Source: CAD feature listing. Evaluate the final solid. Frame: model axes, mm. Face numbers are marked on the shaded views. A direction names the side the tool comes from. Round coordinates to 2 decimals unless told otherwise and drop trailing zeros. Write each loop counter-clockwise with the first axis right and the second up, starting at its lowest first coordinate (ties: lowest second). Pieces come first, ordered by that corner, then holes.
from build123d import *

# Parameters (mm, degrees)
SKETCH_1_R          = 1.5
EXTRUDE_1_DEPTH     = 1.8
EXTRUDE_2_DEPTH     = 2
SKETCH_3_W          = 7.75
SKETCH_3_H          = 0.5
CUT_EXTRUDE_1_DEPTH = 20.686607123


with BuildPart() as part:
    # 草图1 → 凸台-拉伸1 (new body)
    with BuildSketch(Plane.XY):
        with BuildLine():
            Line((-9.503288904, -4.75), (-19, -4.75))
            Line((-19, -4.75), (-19, 4.75))
            Line((-19, 4.75), (19, 4.75))
            Line((19, 4.75), (19, -4.75))
            Line((19, -4.75), (9.503288904, -4.75))
            ThreePointArc((9.503288904, -4.75), (0, -0.5), (-9.503288904, -4.75))
        make_face()
        with Locations((-16, 0.25)):
            Circle(SKETCH_1_R, mode=Mode.SUBTRACT)
        with Locations((16, 0.25)):
            Circle(SKETCH_1_R, mode=Mode.SUBTRACT)
    extrude(amount=EXTRUDE_1_DEPTH)

    # 草图2 → 凸台-拉伸2 (add)
    with BuildSketch(Plane.XY.offset(1.8)):
        with BuildLine():
            Line((-11.25, 4.75), (-11.25, -4.75))
            Line((-11.25, -4.75), (-9.503288904, -4.75))
            ThreePointArc((-9.503288904, -4.75), (0, -0.5), (9.503288904, -4.75))
            Line((9.503288904, -4.75), (11.25, -4.75))
            Line((11.25, -4.75), (11.25, 4.75))
            Line((11.25, 4.75), (-11.25, 4.75))
        make_face()
    extrude(amount=EXTRUDE_2_DEPTH)

    # 草图3 → 切除-拉伸1 (cut, through all)
    with BuildSketch(Plane.XY.offset(1.8)):
        with Locations((-15.125, -4.5)):
            Rectangle(SKETCH_3_W, SKETCH_3_H)
        with Locations((15.125, -4.5)):
            Rectangle(SKETCH_3_W, SKETCH_3_H)
    extrude(amount=-CUT_EXTRUDE_1_DEPTH, mode=Mode.SUBTRACT)


solid = part.part
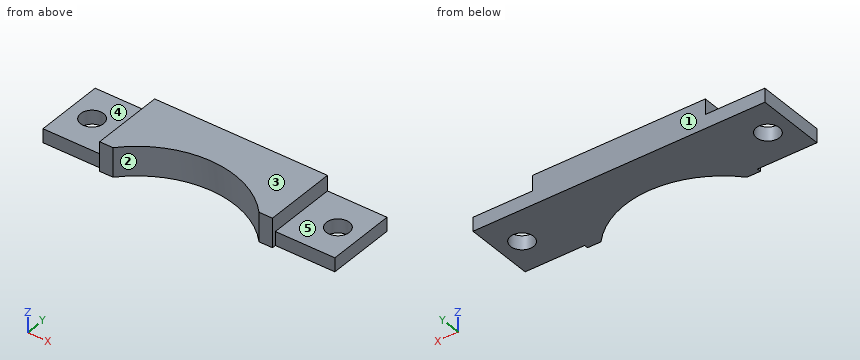
1) Contact query for flat-ended pins moving along their axis: P1, Ø2, axis at x = 14, z = 1, coming from the -Y side; P2, Ø4, axis at x = 17, y = -0.5, coming from the +Z side; P3, Ø1.1, axis at y = 1.5, z = 2.5, coming from the +X side. Output: stop coordinate, or through.
Taken from the geometry:
P1: stops at y = -4.25
P2: stops at z = 1.8
P3: stops at x = 11.25
2) Section query D-D on y = -3.5. Return the cut outline in (x, z).
Taken from the geometry:
outline: (-19, 0) - (-8.22, 0) - (-8.22, 3.8) - (-11.25, 3.8) - (-11.25, 1.8) - (-19, 1.8) - close; (8.22, 0) - (19, 0) - (19, 1.8) - (11.25, 1.8) - (11.25, 3.8) - (8.22, 3.8) - close
3) Section query C-C on z = 0.35. Return the cut outline in (x, y), then the cut area to 3 significant figures.
Taken from the geometry:
outline: (-19, -4.25) - (-11.25, -4.25) - (-11.25, -4.75) - (-9.5, -4.75) arc R12.75 cw to (9.5, -4.75) - (11.25, -4.75) - (11.25, -4.25) - (19, -4.25) - (19, 4.75) - (-19, 4.75) - close; hole circle Ø3 at (-16, 0.25); hole circle Ø3 at (16, 0.25)
area: 283 mm2
4) Section query A-A on y = 0.25. Return the cut outline in (x, z).
Taken from the geometry:
outline: (-19, 0) - (-17.5, 0) - (-17.5, 1.8) - (-19, 1.8) - close; (-14.5, 0) - (14.5, 0) - (14.5, 1.8) - (11.25, 1.8) - (11.25, 3.8) - (-11.25, 3.8) - (-11.25, 1.8) - (-14.5, 1.8) - close; (17.5, 0) - (19, 0) - (19, 1.8) - (17.5, 1.8) - close
5) Pull-direction query (X, two-part tool) for the marked faces 1 and 2; classes: released by +X, released by -X, zero draft, split by the parting line, or undercut.
Taken from the geometry:
face 1: zero draft
face 2: undercut
6) Material intervals for line 1 (Y direction, x = 16, z = 1.4); line 2 (X direction, y = -2.25, z = 0.25); line 3 (Z direction, x = 15, y = -1.25), sorted ascending.
Taken from the geometry:
line 1: y = -4.25 to -1.25, 1.75 to 4.75
line 2: x = -19 to -6.45, 6.45 to 19
line 3: z = 0 to 1.8
7) Section query B-B on x = 15.5. Return the cut outline in (y, z).
Taken from the geometry:
outline: (-4.25, 0) - (-1.16, 0) - (-1.16, 1.8) - (-4.25, 1.8) - close; (1.66, 0) - (4.75, 0) - (4.75, 1.8) - (1.66, 1.8) - close
8) Reachability of the marked faces 3, 4 and 5 from +Z, -Z, +X, -X, +Y, -Y: full face, straight path, thin tool, end or side. Return the list, or none.
Taken from the geometry:
face 3: +Z, +X, -X, +Y, -Y
face 4: +Z, -X, +Y, -Y
face 5: +Z, +X, +Y, -Y
